Read the model definition and answer for the solid it produces. Units are mm, in the model's axes. A direction names the side the tool comes from. Give positions to 0.01 mm unless a question says otherwise; leave off trailing zeros. Order: outer loops, then holes, each group sorted by start corner. A loop starts at its lowest first (then second) coordinate and runs counter-clockwise, first axis right, second up. Notation, with made-up numbers: (28, 39.5) - (72, 39.5) arc R32 cw to (72, 67.5) - close; hole circle Ø8 at (88, 70). An arc over 180 degrees is marked (long way). Return JSON: item names as keys, results as strings.
Autodesk Inventor part; units mm, degrees
ref_plane "YZ Plane" through (0, 0, 0) normal (1, 0, 0) x (0, 1, 0)
ref_plane "XZ Plane" through (0, 0, 0) normal (0, 1, 0) x (-1, 0, 0)
ref_plane "XY Plane" through (0, 0, 0) normal (0, 0, 1) x (1, 0, 0)
sketch "Sketch1" plane through (0, 0, 0) normal (0, 1, 0) x (-1, 0, 0)
  circle A0 centre (0, 0) radius 2
  dimension "d0" = 4
extrude "Extrusion1" add sketch "Sketch1" along normal blind 20
sketch "Sketch2" plane through (0, 20, 0) normal (0, 1, 0) x (1, 0, 0)
  circle A0 centre (0, 0) radius 1.5
  dimension "d3" = 3
extrude "Extrusion2" add sketch "Sketch2" along normal blind 4
sketch "Sketch3" plane through (0, 24, 0) normal (0, 1, 0) x (1, 0, 0)
  line L0 (-1.4497, 0) -> (-0.7249, 1.2555)
  line L1 (-0.7249, 1.2555) -> (0.7249, 1.2555)
  line L2 (0.7249, 1.2555) -> (1.4497, 0)
  line L3 (1.4497, 0) -> (0.7249, -1.2555)
  line L4 (0.7249, -1.2555) -> (-0.7249, -1.2555)
  line L5 (-0.7249, -1.2555) -> (-1.4497, 0)
  point P0 (0, 0)
  point P1 (0, 0)
  dimension "d6" = 2.511
extrude "Extrusion3" add sketch "Sketch3" along normal blind 6
sketch "Sketch4" plane through (0, 30, 0) normal (0, 1, 0) x (1, 0, 0)
  circle A0 centre (0, 0) radius 0.3
  dimension "d9" = 0.6
extrude "Extrusion4" cut sketch "Sketch4" against normal blind 8
properties part number "39-10-202-A2"
Q1. A cutting plane is placed at C-C (y = 20.5). Write down the section's boundary in (x, z).
Values:
{"outline": "circle Ø3 at (0, 0)"}
Q2. A cutting plane is placed at B-B (y = 13.75). Write down the section's boundary in (x, z), and give its area (3 significant figures).
Values:
{"outline": "circle Ø4 at (0, 0)", "area": "12.6 mm²"}
Q3. A cutting plane is placed at A-A (x = 0). Write down the section's boundary in (y, z), and give its area (3 significant figures).
Values:
{"outline": "(0, -2) - (20, -2) - (20, -1.5) - (24, -1.5) - (24, -1.26) - (30, -1.26) - (30, -0.3) - (22, -0.3) - (22, 0.3) - (30, 0.3) - (30, 1.26) - (24, 1.26) - (24, 1.5) - (20, 1.5) - (20, 2) - (0, 2) - close", "area": "102 mm²"}
Q4. Consider L1, parallel to Z at x = 0, y = 27; L2, parallel to Z at x = 0.15, y = 13; L3, parallel to Y at x = -1.45, z = 0.55. Determine where each line is inside the solid, lowest interval first.
Values:
{"L1": "z = -1.26 to -0.3, 0.3 to 1.26", "L2": "z = -1.99 to 1.99", "L3": "y = 0 to 20"}
Q5. Given pin 1 (0.7 mm diameter, centred on x = -0.5, y = 25.5, fed in from -Z); pin 2 (1.6 mm diameter, centred on x = 0, y = 27.5, fed in from +Z), each flat-ended and moving along its own axis, determine where each tip first touches the part or whether it passes through.
Values:
{"pin 1": "stops at z = -1.26", "pin 2": "stops at z = 1.26"}
Q6. For faces 1 (the cylindrical face through (-1.5, 21.97, 0.07)), 2 (the flat face through (1.08, 26.96, -0.64)), 3 (the flat face through (-1.09, 26.96, -0.62)), 4 (the flat face through (0, 27, 1.256)), determine the directions among +Z, -Z, +X, -X, +Y, -Y from which every point of the face is accessible in a straight line to the end or side of a thin tool.
Values:
{"face 1": "+Y", "face 2": "-Z, +X, +Y", "face 3": "-Z, -X, +Y", "face 4": "+Z, +X, -X, +Y"}
